```python
from build123d import *

# Parameters (mm, degrees)
F0_W     = 60
F0_H     = 50
F1_DEPTH = 20
F2_DEPTH = 50
F3_R     = 5
F4_R     = 5
F5_R     = 5
F6_R     = 5
F7_R     = 5


with BuildPart() as f1:
    # F0 (on Top) → F1 (new body)
    with BuildSketch(Plane.XY):
        with Locations((-42, 44.3040782763)):
            Rectangle(F0_W, F0_H)
    extrude(amount=F1_DEPTH)

    # F0 (on Top) → F2 (join)
    with BuildSketch(Plane.XY):
        Polygon((8, 69.3040782763), (-12, 69.3040782763), (-12, 19.3040782763), (8, 19.3040782763), (8, 29.3040782763), (0, 29.3040782763), (0, 59.3040782763), (8, 59.3040782763), align=None)
    extrude(amount=F2_DEPTH)

    # F3
    f3_edges = [f1.edges().sort_by_distance(p)[0] for p in [
        (-72, 44.304078, 20),
    ]]
    fillet(f3_edges, radius=F3_R)

    # F4
    f4_edges = [f1.edges().sort_by_distance(p)[0] for p in [
        (-12, 44.304078, 50),
    ]]
    fillet(f4_edges, radius=F4_R)

    # F5
    f5_edges = [f1.edges().sort_by_distance(p)[0] for p in [
        (-72, 69.304078, 7.5),
        (-72, 44.304078, 15),
        (-72, 44.304078, 0),
        (-72, 19.304078, 7.5),
    ]]
    fillet(f5_edges, radius=F5_R)

    # F6
    f6_edges = [f1.edges().sort_by_distance(p)[0] for p in [
        (8, 24.304078, 50),
        (8, 64.304078, 50),
    ]]
    fillet(f6_edges, radius=F6_R)

    # F7
    f7_edges = [f1.edges().sort_by_distance(p)[0] for p in [
        (8, 24.304078, 0),
        (8, 64.304078, 0),
    ]]
    fillet(f7_edges, radius=F7_R)


solid = f1.part
```
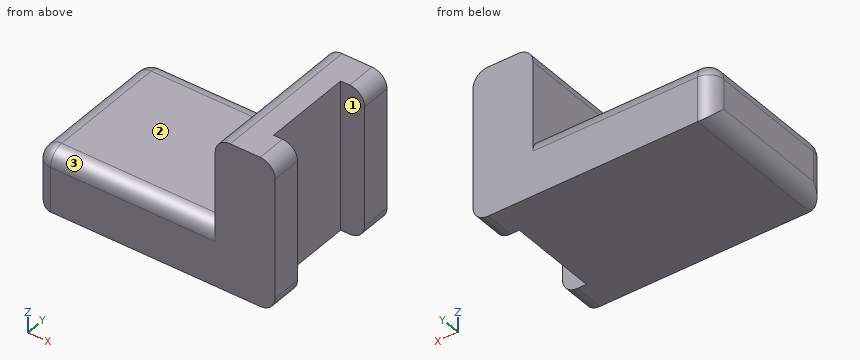
Read the model definition and answer for the solid it produces. Units are mm, in the model's axes. Face numbers are marked on the shaded views. A direction names the side the tool comes from. Give positions to 0.01 mm unless a question says otherwise; leave off trailing zeros. Order: outer loops, then holes, each group sorted by start corner. A loop starts at its lowest first (then second) coordinate and runs counter-clockwise, first axis right, second up.
(1) Find section A-A (x = 2). Give the vertices of the cut face in (y, z).
(2) Straight lines are drawn through the part: L1, parallel to Y at x = 3.5, z = 9.5; L2, parallel to Z at x = -23, y = 51; L3, parallel to X at y = 47, z = 23.5. For each, find the intervals that lie inside material, in ascending order.
(3) Find section D-D (x = -38). Give the vertices of the cut face in (y, z), plus the area to 3 significant figures.
(4) Given pin 1 (2 mm diameter, centred on x = -31.5, y = 25, fed in from +Z); pin 2 (2 mm diameter, centred on y = 37.5, z = 38.5, fed in from +X), each flat-ended and moving along its own axis, determine where each tip first touches the part or whether it passes through.
(5) Find section B-B (y = 36). Give the vertices of the cut face in (x, z).
(6) Find section C-C (z = 7). Give the vertices of the cut face in (x, y).
(7) For the marked faces 1, 2 and 3, determine the directions among +Z, -Z, +X, -X, +Y, -Y from which every point of the face is accessible in a straight line to the end or side of a thin tool.
Result sheet:
1. outline: (19.3, 0) - (29.3, 0) - (29.3, 50) - (19.3, 50) - close; (59.3, 0) - (69.3, 0) - (69.3, 50) - (59.3, 50) - close
2. L1: y = 19.3 to 29.3, 59.3 to 69.3
2. L2: z = 0 to 20
2. L3: x = -12 to 0
3. outline: (19.3, 0) - (69.3, 0) - (69.3, 15) arc R5 ccw to (64.3, 20) - (24.3, 20) arc R5 ccw to (19.3, 15) - close
3. area: 989 mm2
4. pin 1: stops at z = 20
4. pin 2: stops at x = 0
5. outline: (-72, 5) arc R5 ccw to (-67, 0) - (0, 0) - (0, 50) - (-7, 50) arc R5 ccw to (-12, 45) - (-12, 20) - (-67, 20) arc R5 ccw to (-72, 15) - close
6. outline: (-72, 24.3) arc R5 ccw to (-67, 19.3) - (8, 19.3) - (8, 29.3) - (0, 29.3) - (0, 59.3) - (8, 59.3) - (8, 69.3) - (-67, 69.3) arc R5 ccw to (-72, 64.3) - close
7. face 1: +Z, -Z, +X
7. face 2: +Z, -X, +Y, -Y
7. face 3: +Z, -X, -Y
